Study the drawing (mm; zero at the part's minimum x, y, z) and answer. Give positions to 0.01 mm unless a question says otherwise; leave off trailing zeros. Loops run counter-clockwise (first coordinate to the right, second up) from the corner with the lowest first, then second, coordinate; pieces in that order, holes last. Notation, with made-up numbers: (64.5, -13) - (114.5, -13) arc R4 cw to (114.5, -6) - close; hole circle Ø1 at (30.25, 9.5). An arc over 180 degrees is marked (long way). Use one line per item in the form item = value. Start each with the question number.
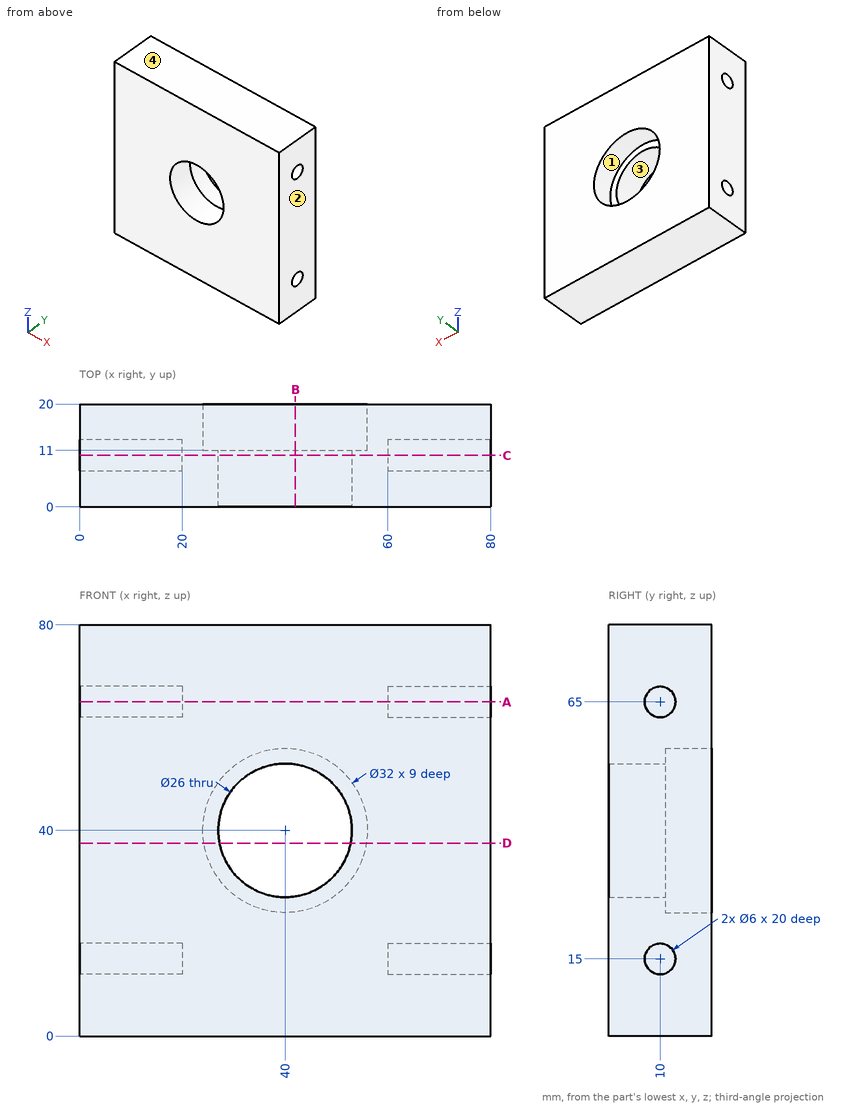
1) Determine the mould class of the marked faces 1, 2, 3 and 4 for opening direction Z: released by +Z, released by -Z, zero draft, split by the parting line, or undercut.
2) A cutting plane is placed at B-B (x = 42). Give the vertices of the cut face in (y, z).
3) A cutting plane is placed at D-D (z = 37.5). Give the vertices of the cut face in (x, y), plus the area to 3 significant figures.
4) Find the intervals of material crossed by probe 1 along Z at (x, y) = (7.25, 10); probe 2 along Z at (x, y) = (16, 9.25); probe 3 along Z at (x, y) = (50, 10.5), in increasing order.
5) Flat-ended cylindrical pins translate along their axes: pin 1 Ø15.5 at (x, z) = (40, 40) entering from +Y; pin 2 Ø8 at (x, z) = (12.5, 69) entering from -Y; pin 3 Ø5.5 at (y, z) = (10, 15) entering from +X; pin 4 Ø1.8 at (y, z) = (11, 64.5) entering from -X. Find the tip coordinate at first contact, or state that the pin passes through.
6) A cutting plane is placed at C-C (y = 10). Give the vertices of the cut face in (x, z), plus the area to 3 significant figures.
7) A cutting plane is placed at A-A (z = 65). Give the vertices of the cut face in (x, y), plus the area to 3 significant figures.
Answer sheet:
q1.face_1 = undercut
q1.face_2 = zero draft
q1.face_3 = undercut
q1.face_4 = released by +Z
q2.outline = (0, 0) - (20, 0) - (20, 24.13) - (11, 24.13) - (11, 27.15) - (0, 27.15) - close; (0, 52.85) - (11, 52.85) - (11, 55.87) - (20, 55.87) - (20, 80) - (0, 80) - close
q3.outline = (0, 0) - (27.24, 0) - (27.24, 11) - (24.2, 11) - (24.2, 20) - (0, 20) - close; (52.76, 0) - (80, 0) - (80, 20) - (55.8, 20) - (55.8, 11) - (52.76, 11) - close
q3.area = 1,030 mm²
q4.probe_1 = 0 to 12, 18 to 62, 68 to 80
q4.probe_2 = 0 to 12.1, 17.9 to 62.1, 67.9 to 80
q4.probe_3 = 0 to 31.69, 48.31 to 80
q5.pin_1 = through
q5.pin_2 = 0
q5.pin_3 = 60
q5.pin_4 = 20
q6.outline = (0, 0) - (80, 0) - (80, 12) - (60, 12) - (60, 18) - (80, 18) - (80, 62) - (60, 62) - (60, 68) - (80, 68) - (80, 80) - (0, 80) - (0, 68) - (20, 68) - (20, 62) - (0, 62) - (0, 18) - (20, 18) - (20, 12) - (0, 12) - close; hole circle Ø26 at (40, 40)
q6.area = 5,390 mm²
q7.outline = (0, 0) - (80, 0) - (80, 7) - (60, 7) - (60, 13) - (80, 13) - (80, 20) - (0, 20) - (0, 13) - (20, 13) - (20, 7) - (0, 7) - close
q7.area = 1,360 mm²
